Autodesk Inventor part; units mm, degrees
ref_plane "YZ Plane" through (0, 0, 0) normal (1, 0, 0) x (0, 1, 0)
ref_plane "XZ Plane" through (0, 0, 0) normal (0, 1, 0) x (-1, 0, 0)
ref_plane "XY Plane" through (0, 0, 0) normal (0, 0, 1) x (1, 0, 0)
sketch "Esboço1" plane through (0, 0, 0) normal (0, 0, 1) x (1, 0, 0)
  circle A0 centre (0, 0) radius 3.75
  circle A1 centre (0, 0) radius 7.2
  circle A2 centre (0, 0) radius 9.2
  dimension "d0" = 7.5
  dimension "d2" = 14.4
  dimension "d3" = 18.4
extrude "Extrusão1" add sketch "Esboço1" along normal blind 7 contours A1 | A2
sketch "Esboço2" plane through (0, 0, 7) normal (0, 0, 1) x (1, 0, 0)
  circle A0 centre (0, 0) radius 9.2
  line L0 (-9.2, 1.9) -> (-9.2, -1.9)
  line L1 (-1.9, 9.2) -> (1.9, 9.2)
  line L2 (9.2, 1.9) -> (9.2, -1.9)
  line L3 (-1.9, -9.2) -> (1.9, -9.2)
  line L4 (-1.9, 9.2) -> (-1.9, 3.1165)
  line L5 (-1.9, -3.1165) -> (-1.9, -9.2)
  line L6 (1.9, 9.2) -> (1.9, 3.1165)
  line L7 (1.9, -3.1165) -> (1.9, -9.2)
  line L8 (-9.2, -1.9) -> (-3.1165, -1.9)
  line L9 (3.1165, -1.9) -> (9.2, -1.9)
  line L10 (-9.2, 1.9) -> (-3.1165, 1.9)
  line L11 (3.1165, 1.9) -> (9.2, 1.9)
  arc A1 (-3.1165, -1.9) -> (-1.9, -3.1165) centre (0, 0) ccw
  arc A2 (1.9, -3.1165) -> (3.1165, -1.9) centre (0, 0) ccw
  arc A3 (3.1165, 1.9) -> (1.9, 3.1165) centre (0, 0) ccw
  arc A4 (-1.9, 3.1165) -> (-3.1165, 1.9) centre (0, 0) ccw
  point P0 (9.0017, 1.9)
  point P1 (1.9, 9.0017)
  point P2 (1.9, -9.0017)
  point P3 (9.0017, -1.9)
  point P4 (-9.0017, -1.9)
  point P5 (-1.9, -9.0017)
  point P6 (-1.9, 9.0017)
  point P7 (-9.0017, 1.9)
extrude "Extrusão2" cut sketch "Esboço2" against normal blind 3.2 contours L11 A3 L6 A0 | A0 L7 A2 L9 | L4 A4 L10 A0 | A0 L8 A1 L5
fillet "Arredondamento1" radius 0.5 9 edges at (-3.75, 0, 7) (0, 3.75, 7) (3.6185, -0.9845, 7) (3.6185, 0.9845, 7) (0, -3.75, 7) (-2.6517, -2.6517, 3.8) (-2.6517, 2.6517, 3.8) (2.6517, 2.6517, 3.8) (2.6517, -2.6517, 3.8)
properties part number "trava_botao_topo_3DPrint"
For this review, take the finished solid that the model builds, in its own axes (mm). A direction names the side the tool comes from. Round coordinates to 2 decimals unless told otherwise and drop trailing zeros. Write each loop counter-clockwise with the first axis right and the second up, starting at its lowest first coordinate (ties: lowest second). Pieces come first, ordered by that corner, then holes. Notation, with made-up numbers: (38.25, -20) -> (88.25, -20) arc R21 cw to (88.25, -10) -> close; hole circle Ø11 at (46.5, 41.5). An arc over 180 degrees is marked (long way). One line per question, with ' | ' between items. Start each with the question number.
(1) Tool access review of faces 1 (the face through (5, -5, 3.8)), 2 (the face through (-5, 5, 3.8)), 3 (the face through (5, 5, 3.8)), 4 (the face through (-5, -5, 3.8)), 5 (the face through (-6.78, -6.22, 2.67)): name each direction out of +Z, -Z, +X, -X, +Y, -Y from which nothing blocks a thin tool from reaching the whole face with its end or side.
(2) Add section B-B, the plane x = 0. Write out the cut boundary in (y, z), plus the area to 3 significant figures.
(3) Add section A-A, the plane z = 6.25. Write out the cut boundary in (x, y).
(4) Add section D-D, the plane z = 1.25. Write out the cut boundary in (x, y), plus the area to 3 significant figures.
(5) Insertion check: P1, Ø5.5, axis at x = -6.5, y = -7, coming from the +Z side; P2, Ø2, axis at x = 2, z = 2, coming from the -Y side; P3, Ø3, axis at y = -7, z = 6, coming from the +X side. Each pin has a flat end and moves straight along its axis. Give the tip position at first contact, or say it passes through.
(6) For line 1 along Y through (x, z) = (0, 6.5); line 2 along Z through (x, y) = (5.25, -5); line 3 along Y through (x, z) = (-7.5, 6.75), list the stretches that pass through material, from the lowest coordinate up. Write a range as from..to.
Answer list:
1) face 1: +Z, +X, -Y | face 2: +Z, -X, +Y | face 3: +Z, +X, +Y | face 4: +Z, -X, -Y | face 5: +Z, -Z
2) outline: (-9.2, 0) -> (-3.75, 0) -> (-3.75, 6.5) arc R0.5 ccw to (-4.25, 7) -> (-9.2, 7) -> close; (3.75, 0) -> (9.2, 0) -> (9.2, 7) -> (4.25, 7) arc R0.5 ccw to (3.75, 6.5) -> close | area: 76.2 mm²
3) outline: (-9, -1.9) -> (-3.23, -1.9) arc R3.75 cw to (-3.23, 1.9) -> (-9, 1.9) arc R9.2 ccw to start; (-1.9, -9) arc R9.2 ccw to (1.9, -9) -> (1.9, -3.23) arc R3.75 cw to (-1.9, -3.23) -> close; (-1.9, 3.23) arc R3.75 cw to (1.9, 3.23) -> (1.9, 9) arc R9.2 ccw to (-1.9, 9) -> close; (3.23, -1.9) -> (9, -1.9) arc R9.2 ccw to (9, 1.9) -> (3.23, 1.9) arc R3.75 cw to start
4) outline: circle Ø18.4 at (0, 0); hole circle Ø7.5 at (0, 0) | area: 222 mm²
5) P1: z = 3.8 | P2: y = -9.15 | P3: x = 1.9
6) line 1: -9.2..-3.75, 3.75..9.2 | line 2: 0..3.8 | line 3: -1.9..1.9
